```python
from build123d import *

# Parameters (mm, degrees)
BOSS_EXTRUDE1_DEPTH  = 87.3
CUT_EXTRUDE1_REACH   = 7
SKETCH2_R            = 2.5
SKETCH3_W            = 75.3
SKETCH3_H            = 16.36
CUT_EXTRUDE2_DEPTH   = 19.693329973
SKETCH4_W            = 2
SKETCH4_H            = 12
SKETCH4_H_2          = 22
BOSS_EXTRUDE2_DEPTH  = 87.3
BOSS_EXTRUDE16_DEPTH = 2
LPATTERN1_COUNT      = 2
LPATTERN1_PITCH      = 89.3
CUT_EXTRUDE4_DEPTH   = 0.5
CUT_EXTRUDE5_DEPTH   = 0.5
SKETCH14_W           = 88.3
SKETCH14_H           = 8.306670027
CUT_EXTRUDE6_DEPTH   = 0.5
SKETCH15_W           = 88.3
SKETCH15_H           = 8.482653923
CUT_EXTRUDE7_DEPTH   = 0.5


with BuildPart() as part:
    # Sketch1 → Boss-Extrude1 (new body)
    with BuildSketch(Plane(origin=(0, 0, 0), x_dir=(0, 0, -1), z_dir=(1, 0, 0))):
        Polygon((-73.551459735, 26.94681652), (-43.711459735, 40.640146493), (-43.711459735, 26.94681652), (-31.711459735, 26.94681652), (-31.711459735, 21.94681652), (-113.911459735, 21.94681652), (-113.911459735, 26.94681652), (-101.911459735, 26.94681652), (-101.911459735, 30.464162597), align=None)
    extrude(amount=BOSS_EXTRUDE1_DEPTH)

    # Sketch2 → Cut-Extrude1 (cut, up to next)
    with BuildSketch(Plane(origin=(0, 26.94681652, 0), x_dir=(1, 0, 0), z_dir=(0, 1, 0)), mode=Mode.PRIVATE) as cut_extrude1_sk1:
        with Locations((15, -36.711459735)):
            Circle(SKETCH2_R)
    cut_extrude1_tool1 = extrude(cut_extrude1_sk1.sketch, amount=-CUT_EXTRUDE1_REACH, mode=Mode.PRIVATE) & part.part
    add(cut_extrude1_tool1.solids().sort_by_distance((15, 26.946817, 36.71146))[0], mode=Mode.SUBTRACT)
    # Sketch2 → Cut-Extrude1 (cut, up to next)
    with BuildSketch(Plane(origin=(0, 26.94681652, 0), x_dir=(1, 0, 0), z_dir=(0, 1, 0)), mode=Mode.PRIVATE) as cut_extrude1_sk2:
        with Locations((72.333370453, -36.711459735)):
            Circle(SKETCH2_R)
    cut_extrude1_tool2 = extrude(cut_extrude1_sk2.sketch, amount=-CUT_EXTRUDE1_REACH, mode=Mode.PRIVATE) & part.part
    add(cut_extrude1_tool2.solids().sort_by_distance((72.33337, 26.946817, 36.71146))[0], mode=Mode.SUBTRACT)
    # Sketch2 → Cut-Extrude1 (cut, up to next)
    with BuildSketch(Plane(origin=(0, 26.94681652, 0), x_dir=(1, 0, 0), z_dir=(0, 1, 0)), mode=Mode.PRIVATE) as cut_extrude1_sk3:
        with Locations((72.333370453, -108.911459735)):
            Circle(SKETCH2_R)
    cut_extrude1_tool3 = extrude(cut_extrude1_sk3.sketch, amount=-CUT_EXTRUDE1_REACH, mode=Mode.PRIVATE) & part.part
    add(cut_extrude1_tool3.solids().sort_by_distance((72.33337, 26.946817, 108.91146))[0], mode=Mode.SUBTRACT)
    # Sketch2 → Cut-Extrude1 (cut, up to next)
    with BuildSketch(Plane(origin=(0, 26.94681652, 0), x_dir=(1, 0, 0), z_dir=(0, 1, 0)), mode=Mode.PRIVATE) as cut_extrude1_sk4:
        with Locations((15, -108.911459735)):
            Circle(SKETCH2_R)
    cut_extrude1_tool4 = extrude(cut_extrude1_sk4.sketch, amount=-CUT_EXTRUDE1_REACH, mode=Mode.PRIVATE) & part.part
    add(cut_extrude1_tool4.solids().sort_by_distance((15, 26.946817, 108.91146))[0], mode=Mode.SUBTRACT)

    # Sketch3 → Cut-Extrude2 (cut, through all)
    with BuildSketch(Plane.XZ.offset(-21.94681652)):
        with Locations((43.65, 87.731459735)):
            Rectangle(SKETCH3_W, SKETCH3_H)
        with Locations((43.65, 59.371459735)):
            Rectangle(SKETCH3_W, SKETCH3_H)
    extrude(amount=-CUT_EXTRUDE2_DEPTH, mode=Mode.SUBTRACT)

    # Sketch4 → Boss-Extrude2 (add, through all)
    with BuildSketch(Plane(origin=(87.3, 0, 0), x_dir=(0, 0, -1), z_dir=(1, 0, 0))):
        with Locations((-102.911459735, 32.94681652)):
            Rectangle(SKETCH4_W, SKETCH4_H)
        with Locations((-42.711459735, 37.94681652)):
            Rectangle(SKETCH4_W, SKETCH4_H_2)
    extrude(amount=-BOSS_EXTRUDE2_DEPTH)

    # Sketch8 → Boss-Extrude16 (add)
    with BuildSketch(Plane(origin=(87.3, 0, 0), x_dir=(0, 0, -1), z_dir=(1, 0, 0))):
        Polygon((-103.911459735, 38.94681652), (-101.911459735, 38.94681652), (-43.711459735, 48.94681652), (-41.711459735, 48.94681652), (-41.711459735, 26.94681652), (-31.711459735, 26.94681652), (-31.711459735, 21.94681652), (-113.911459735, 21.94681652), (-113.911459735, 26.94681652), (-103.911459735, 26.94681652), align=None)
    boss_extrude16 = extrude(amount=BOSS_EXTRUDE16_DEPTH)

    # LPattern1: Boss-Extrude16 ×2
    with Locations(*[(-i * LPATTERN1_PITCH, 0, 0) for i in range(1, LPATTERN1_COUNT)]):
        add(boss_extrude16)

    # Sketch12 → Cut-Extrude4 (cut)
    with BuildSketch(Plane(origin=(0, 0, 0), x_dir=(0, 0, -1), z_dir=(1, 0, 0))):
        Polygon((-43.711459735, 48.94681652), (-43.711459735, 40.640146493), (-73.551459735, 26.94681652), (-101.911459735, 30.464162597), (-101.911459735, 38.94681652), align=None)
    extrude(amount=-CUT_EXTRUDE4_DEPTH, mode=Mode.SUBTRACT)

    # Sketch13 → Cut-Extrude5 (cut)
    with BuildSketch(Plane.ZY.offset(-87.3)):
        Polygon((43.711459735, 40.640146493), (43.711459735, 48.94681652), (101.911459735, 38.94681652), (101.911459735, 30.464162597), (73.551459735, 26.94681652), align=None)
    extrude(amount=-CUT_EXTRUDE5_DEPTH, mode=Mode.SUBTRACT)

    # Sketch14 → Cut-Extrude6 (cut)
    with BuildSketch(Plane.XY.offset(43.711459735)):
        with Locations((43.65, 44.793481507)):
            Rectangle(SKETCH14_W, SKETCH14_H)
    extrude(amount=-CUT_EXTRUDE6_DEPTH, mode=Mode.SUBTRACT)

    # Sketch15 → Cut-Extrude7 (cut)
    with BuildSketch(Plane(origin=(0, 0, 101.911459735), x_dir=(-1, 0, 0), z_dir=(0, 0, -1))):
        with Locations((-43.65, 34.705489559)):
            Rectangle(SKETCH15_W, SKETCH15_H)
    extrude(amount=-CUT_EXTRUDE7_DEPTH, mode=Mode.SUBTRACT)


solid = part.part
```
Could you check a few things on this model? Use its own coordinates, in mm. A direction names the side the tool comes from. Give positions to 0.01 mm unless a question says otherwise; leave off trailing zeros. Write each loop counter-clockwise with the first axis right and the second up, starting at its lowest first coordinate (ties: lowest second). Pieces come first, ordered by that corner, then holes. Notation, with made-up numbers: (-25.5, -21.5) -> (-4.5, -21.5) arc R18 ccw to (-4.5, 9.5) -> close; hole circle Ø7 at (71.25, 32). An arc over 180 degrees is marked (long way). Write each question's results on one line, items separated by ' | '.
1. I want a section at B-B, the plane z = 81. Write out the boundary of the cut face in (x, y).
Check sheet entries:
outline: (-2, 21.95) -> (6, 21.95) -> (6, 27.87) -> (-0.5, 27.87) -> (-0.5, 42.54) -> (-2, 42.54) -> close; (81.3, 21.95) -> (89.3, 21.95) -> (89.3, 42.54) -> (87.8, 42.54) -> (87.8, 27.87) -> (81.3, 27.87) -> close
2. On a 3-axis mill with a long thin cutter (end or side, diameter ignored), from which of +Z, -Z, +X, -X, +Y, -Y can I reach the whole of each face in a straight line? I mean faces 4 (the flat face through (43, 45, 43.211)), 5 (the flat face through (43, 38.947, 103)), 6 (the flat face through (43.03, 29.13, 68.79)), 7 (the flat face through (43, 26, 67.551)), 8 (the flat face through (43, 26.947, 37)). Say none if no direction works.
Check sheet entries:
face 4: +Z, +Y | face 5: +Z, +X, -X, +Y | face 6: +Y | face 7: +Y, -Y | face 8: -Z, +X, -X, +Y
3. I want a section at D-D, the plane y = 34.5. Write out the boundary of the cut face in (x, z), then the cut area to 3 significant figures.
Check sheet entries:
outline: (-2, 41.71) -> (89.3, 41.71) -> (89.3, 103.91) -> (-2, 103.91) -> close; hole (-0.5, 57.09) -> (6, 57.09) -> (6, 51.19) -> (81.3, 51.19) -> (81.3, 57.09) -> (87.8, 57.09) -> (87.8, 102.41) -> (-0.5, 102.41) -> close | area: 1,230 mm²
4. I want a section at A-A, the plane x = 55.5. Write out the boundary of the cut face in (y, z), then the cut area to 3 significant figures.
Check sheet entries:
outline: (21.95, 31.71) -> (26.95, 31.71) -> (26.95, 41.71) -> (48.95, 41.71) -> (48.95, 43.21) -> (40.64, 43.21) -> (40.64, 43.71) -> (37.21, 51.19) -> (21.95, 51.19) -> close; (21.95, 67.55) -> (29.7, 67.55) -> (26.95, 73.55) -> (27.69, 79.55) -> (21.95, 79.55) -> close; (21.95, 95.91) -> (29.72, 95.91) -> (30.46, 101.91) -> (30.46, 102.41) -> (38.95, 102.41) -> (38.95, 103.91) -> (26.95, 103.91) -> (26.95, 113.91) -> (21.95, 113.91) -> close | area: 426 mm²
5. I need wall thicknesses on L1, parallel to Z at x = 15, y = 24.25; L2, parallel to X at y = 25, z = 95.5; L3, parallel to X at y = 35.75, z = 86. Which ranges of each line are inside material? Lowest first, please.
Check sheet entries:
L1: z = 31.71 to 34.21, 39.21 to 51.19, 67.55 to 79.55, 95.91 to 106.41, 111.41 to 113.91 | L2: x = -2 to 6, 81.3 to 89.3 | L3: x = -2 to -0.5, 87.8 to 89.3
6. If we mould it in two halves opening along X, with no side actions, what happens to faces 1 (the flat face through (89.3, 33, 72)), 2 (the flat face through (43, 38, 41.711)), 3 (the flat face through (81.3, 25, 88))? For each: released by +X, released by -X, zero draft, split by the parting line, or undercut.
Check sheet entries:
face 1: released by +X | face 2: zero draft | face 3: undercut
7. I want a section at C-C, the plane x = 15. Count the separate pieces of the cut face and the enclosed holes in it, then the cut area to 3 significant figures.
Check sheet entries:
separate pieces: 5 | enclosed holes: 0 | area: 376 mm²
8. Will these pins go through, and if not, where does the flat tip stop? pin 1 Ø1.6 at (x, z) = (56.5, 103) entering from +Y; pin 2 Ø12 at (x, z) = (33.5, 79.5) entering from +Y; pin 3 Ø2 at (x, y) = (58, 29.5) entering from +Z.
Check sheet entries:
pin 1: stops at y = 38.95 | pin 2: stops at y = 27.69 | pin 3: stops at z = 103.91
